Build history of the part. All positions in model axes, mm. Face numbers are marked on the shaded views. Give positions to 0.01 mm unless a question says otherwise; leave off trailing zeros. Loops run counter-clockwise (first coordinate to the right, second up) from the corner with the lowest first, then second, coordinate; pieces in that order, holes last.
1) Band-saw the part on C-C on z = 17. List the corners of the cut face in (x, y).
2) Flat gauge pins, fed straight in: P1, Ø5, axis at x = -1.5, z = 12.5, coming from the +Y side; P2, Ø5, axis at x = 0, y = 4.5, coming from the -Z side; P3, Ø1, axis at y = 5.5, z = 15.5, coming from the +X side. Where does each tip first touch, or does it go through?
3) Wall check: line 1 (Z direction, x = -3.25, y = 5); line 2 (Z direction, x = 3, y = 3.25); line 3 (Y direction, x = -4.25, z = 14.25). Give the ranges that are in metal, low to high.
4) Band-saw the part on A-A on y = 3.75. List the corners of the cut face in (x, z).
5) Two-plate mould, pull along Y, no slides. Class the marked faces 1, 2 and 3: +Y half, -Y half, draft (parallel to the pull), parting line (faces both ways), or undercut.
6) Band-saw the part on D-D on y = 7.5. List the corners of the cut face in (x, z), then the cut area to 3 significant figures.
7) Band-saw the part on B-B on x = -0.5. List the corners of the cut face in (y, z), then the cut area to 3 significant figures.
```python
from build123d import *

# Parameters (mm, degrees)
REVOLVE1_ANGLE            = 45
CUT_EXTRUDE1_DEPTH        = 28.647117169
CUT_EXTRUDE1_DEPTH_BACK   = 28.647117169
CUT_EXTRUDE4_REACH        = 29.998
CUT_EXTRUDE4_START_RADIUS = 14.22
CUT_EXTRUDE4_END_RADIUS   = 14.22
CUT_EXTRUDE5_DEPTH        = 27.866361913
CUT_EXTRUDE5_DEPTH_BACK   = 27.866361913
SKETCH9_R                 = 2.6035


with BuildPart() as part:
    # Sketch1 → Revolve1 (revolve, symmetric)
    with BuildSketch(Plane(origin=(0, 0, 0), x_dir=(0, 0, -1), z_dir=(1, 0, 0))) as revolve1_sk:
        with BuildLine():
            Line((-14.217802221, 0.25), (-19.048359509, 0.25))
            ThreePointArc((-19.048359509, 0.25), (-14.676690222, 12.144845166), (-3.81, 18.66511184))
            Line((-3.81, 18.66511184), (-3.81, 13.700083941))
            ThreePointArc((-3.81, 13.700083941), (-11.246181696, 8.70240181), (-14.217802221, 0.25))
        make_face()
    revolve(axis=Axis((0, 0, 0), (0, 1, 0)), revolution_arc=REVOLVE1_ANGLE / 2)
    revolve(revolve1_sk.sketch, axis=Axis((0, 0, 0), (0, -1, 0)), revolution_arc=REVOLVE1_ANGLE / 2)

    # Sketch2 → Cut-Extrude1 (cut, two sides: drawn at the far end of the back side and taken through both)
    with BuildSketch(Plane(origin=(0, 0, 0), x_dir=(1, 0, 0), z_dir=(0, 1, 0)).offset(-CUT_EXTRUDE1_DEPTH_BACK)):
        with BuildLine():
            Line((7.289491598, -17.598389479), (1.458023877, -3.519981019))
            ThreePointArc((1.458023877, -3.519981019), (1.400077392, -3.543428184), (1.341754023, -3.5659215))
            Line((1.341754023, -3.5659215), (7.173849701, -17.645845983))
            ThreePointArc((7.173849701, -17.645845983), (7.231709577, -17.622212591), (7.289491598, -17.598389479))
        make_face()
        with BuildLine():
            Line((-7.173849701, -17.645845983), (-1.341754023, -3.5659215))
            ThreePointArc((-1.341754023, -3.5659215), (-1.400077392, -3.543428184), (-1.458023877, -3.519981019))
            Line((-1.458023877, -3.519981019), (-7.289491598, -17.598389479))
            ThreePointArc((-7.289491598, -17.598389479), (-7.231709577, -17.622212591), (-7.173849701, -17.645845983))
        make_face()
    extrude(amount=CUT_EXTRUDE1_DEPTH + CUT_EXTRUDE1_DEPTH_BACK, mode=Mode.SUBTRACT)

    # Cut-Extrude4: from a sphere face, 29.998 long prism both ways, kept between that surface and its translate by the depth
    cut_extrude4_start = Location((0, 0, 0)) * Sphere(CUT_EXTRUDE4_START_RADIUS, mode=Mode.PRIVATE)
    cut_extrude4_end = Location((0, 0.145802388, 0.351998102)) * Sphere(CUT_EXTRUDE4_END_RADIUS, mode=Mode.PRIVATE)
    # Sketch8 → Cut-Extrude4 (cut, from a surface)
    with BuildSketch(Plane(origin=(0, 0, 0), x_dir=(-1, 0, 0), z_dir=(0, 0.3826834323650899, 0.9238795325112868)), mode=Mode.PRIVATE) as cut_extrude4_sk1:
        Polygon((-1.253717949, -0.505052528), (1.481666667, -0.505052528), (-0.854807692, 4.053921831), (-1.199402043, 3.864261374), (0.80672476, -0.049155093), (-1.253717949, -0.049155093), align=None)
    cut_extrude4_tool1 = extrude(cut_extrude4_sk1.sketch, amount=CUT_EXTRUDE4_REACH, both=True, mode=Mode.PRIVATE)
    add(((cut_extrude4_tool1 - cut_extrude4_start) & cut_extrude4_end).solids().sort_by_distance((-0.113974, 5.809704, 12.845032))[0], mode=Mode.SUBTRACT)

    # Sketch9 → Cut-Extrude5 (cut, two sides: drawn at the far end of the back side and taken through both)
    with BuildSketch(Plane(origin=(5.827608686, 18.858537854, 17.935535314), x_dir=(-0.8206892018836905, -0.23968096505674552, 0.5186735668038023), z_dir=(-0.2185080122244017, -0.7071067811865477, -0.67249851196396)).offset(-CUT_EXTRUDE5_DEPTH_BACK)):
        Circle(SKETCH9_R)
    extrude(amount=CUT_EXTRUDE5_DEPTH + CUT_EXTRUDE5_DEPTH_BACK, mode=Mode.SUBTRACT)


solid = part.part
```
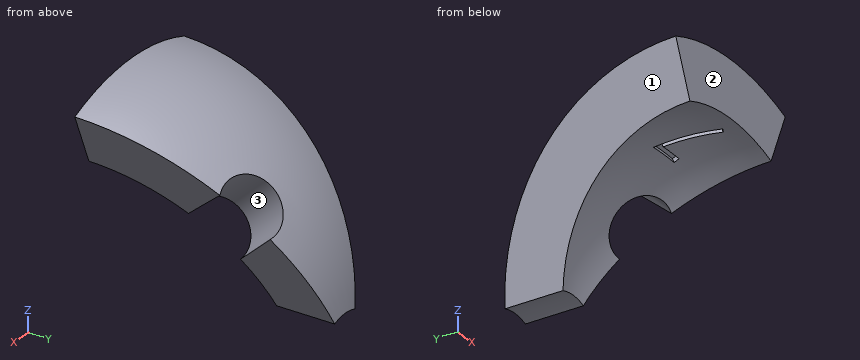
Findings below:
1. outline: (-6.91, 0.25) - (6.91, 0.25) - (6.91, 5.12) arc R8.6 ccw to (-6.91, 5.12) - close
2. P1: stops at y = 16.16
2. P2: stops at z = 12.38
2. P3: stops at x = 6.49
3. line 1: z = 12.91 to 18.09
3. line 2: z = 13.51 to 18.53
3. line 3: y = 0.25 to 11.91
4. outline: (-7.03, 17.3) - (-5.13, 12.72) arc R13.72 cw to (-0.31, 13.71) - (-0.23, 14.11) arc R13.76 cw to (0.21, 14.11) - (0.13, 13.72) arc R13.72 cw to (5.13, 12.72) - (7.03, 17.3) arc R18.68 ccw to start
5. face 1: draft
5. face 2: -Y half
5. face 3: undercut
6. outline: (-6.59, 16.23) - (-4.51, 11.21) arc R12.08 cw to (4.51, 11.21) - (6.59, 16.23) arc R17.51 ccw to start
6. area: 61.7 mm2
7. outline: (0.25, 14.21) arc R14.21 cw to (4.11, 13.6) - (4.25, 13.96) arc R14.21 cw to (5.07, 13.68) - (4.93, 13.33) arc R14.21 cw to (5.48, 13.11) - (5.63, 13.46) arc R14.21 cw to (6.05, 13.28) - (5.9, 12.93) arc R14.21 cw to (13.7, 3.78) - (18.67, 3.78) arc R19.04 ccw to (0.25, 19.04) - close
7. area: 106 mm2
